```python
from build123d import *

# Parameters (mm, degrees)
SKETCH1_R                  = 38.1
BOSS_EXTRUDE1_DEPTH        = 6.35
SKETCH3_R                  = 38.1
SKETCH3_R_2                = 34.8488
CUT_EXTRUDE_THIN1_DEPTH    = 3.175
F_1_2_0_5_DIAMETER_HOLE1_D = 28.575
F_8_32_TAPPED_HOLE1_D      = 3.4544
CIRPATTERN1_COUNT          = 6


with BuildPart() as part:
    # Sketch1 → Boss-Extrude1 (new body)
    with BuildSketch(Plane(origin=(0, 0, 0), x_dir=(0, 0, -1), z_dir=(1, 0, 0))):
        Circle(SKETCH1_R)
    extrude(amount=BOSS_EXTRUDE1_DEPTH)

    # Sketch3 → Cut-Extrude-Thin1 (cut)
    with BuildSketch(Plane(origin=(6.35, 0, 0), x_dir=(0, 0, -1), z_dir=(1, 0, 0))):
        Circle(SKETCH3_R)
        Circle(SKETCH3_R_2, mode=Mode.SUBTRACT)
    extrude(amount=-CUT_EXTRUDE_THIN1_DEPTH, mode=Mode.SUBTRACT)

    # 1/2 (0.5) Diameter Hole1 (through all)
    with Locations(Plane(origin=(6.35, 0, 0), x_dir=(0, 0, -1), z_dir=(1, 0, 0))):
        with Locations((0, 0)):
            Hole(F_1_2_0_5_DIAMETER_HOLE1_D / 2)

    # #8-32 Tapped Hole1 (through all)
    with Locations(Plane.ZY):
        with Locations((0, 23.8125)):
            f_8_32_tapped_hole1 = Hole(F_8_32_TAPPED_HOLE1_D / 2)

    # CirPattern1: #8-32 Tapped Hole1 ×6 about axis
    cirpattern1_axis = Axis((0, 0, 0), (1, 0, 0))
    for i in range(1, CIRPATTERN1_COUNT):
        add(f_8_32_tapped_hole1.rotate(cirpattern1_axis, i * 360 / CIRPATTERN1_COUNT), mode=Mode.SUBTRACT)


solid = part.part
```
Work out the finished part from the listing and answer in its coordinate system (mm). A direction names the side the tool comes from. Round coordinates to 2 decimals unless told otherwise and drop trailing zeros. Loops run counter-clockwise (first coordinate to the right, second up) from the corner with the lowest first, then second, coordinate; pieces in that order, holes last.
(1) Find the intervals of material crossed by L1, parallel to Y at x = 4.5, z = 0; L2, parallel to Z at x = 2.5, y = 11; L3, parallel to Y at x = 5.75, z = -8, in increasing order.
Computed values:
L1: y = -34.85 to -25.54, -22.09 to -14.29, 14.29 to 22.09, 25.54 to 34.85
L2: z = -36.48 to -22.09, -19.15 to -9.12, 9.12 to 19.15, 22.09 to 36.48
L3: y = -33.92 to -11.84, 11.84 to 33.92
(2) The part is cut by section A-A, the plane z = 0. Give the number of separate pieces and of enclosed holes in the cut face, and give its area (3 significant figures).
Computed values:
separate pieces: 4
enclosed holes: 0
area: 238 mm2
(3) For faces 4 (the cylindrical face through (4.785, -21.205, 27.655)), 5 (the cylindrical face through (3.219, -25.525, -0.225)), determine the directions among +Z, -Z, +X, -X, +Y, -Y from which every point of the face is accessible in a straight line to the end or side of a thin tool.
Computed values:
face 4: +X
face 5: +X, -X
(4) The part is cut by section C-C, the plane x = 4.25. Give the vertices of the cut face in (y, z) (1 decimal).
Computed values:
outline: circle Ø69.7 at (0, 0); hole circle Ø3.5 at (-23.8, 0); hole circle Ø28.6 at (0, 0); hole circle Ø3.5 at (-11.9, -20.6); hole circle Ø3.5 at (-11.9, 20.6); hole circle Ø3.5 at (11.9, -20.6); hole circle Ø3.5 at (11.9, 20.6); hole circle Ø3.5 at (23.8, 0)
(5) This flat-tipped pin is pushed along its axis until it touches: P1, Ø3, axis at x = 4, y = 5, coming from the +Z side. Where does it stop, or does it pass through?
Computed values:
P1: stops at z = 37.92
(6) The part is cut by section D-D, the plane z = 8.5. Give the vertices of the cut face in (x, y) (3 decimals).
Computed values:
outline: (0, -37.14) - (3.175, -37.14) - (3.175, -33.796) - (6.35, -33.796) - (6.35, -11.484) - (0, -11.484) - close; (0, 11.484) - (6.35, 11.484) - (6.35, 33.796) - (3.175, 33.796) - (3.175, 37.14) - (0, 37.14) - close
(7) The mould has two halves that part along Z. Classify faces 1 (the cylindrical face through (1.565, -23.183, 30.235)), 2 (the cylindrical face through (3.219, -10.194, -20.397)), 3 (the flat face through (0, 1, -16)): pulls with the +Z half, pulls with the -Z half, needs draft (parallel to the pull), parting line crosses it, or undercut.
Computed values:
face 1: parting line crosses it
face 2: undercut
face 3: needs draft
